The listing builds one solid part. Answer for the finished solid, in the listing's coordinates (mm). A direction names the side the tool comes from. Round coordinates to 2 decimals unless told otherwise and drop trailing zeros. Write each loop counter-clockwise with the first axis right and the second up, starting at its lowest first coordinate (ties: lowest second). Pieces come first, ordered by that corner, then holes.
(1) A cutting plane is placed at D-D, the plane y = -19.5. Give the vertices of the cut face in (x, z), and give its area (3 significant figures).
(2) A cutting plane is placed at B-B, the plane x = 25.5. Give the vertices of the cut face in (y, z).
(3) A cutting plane is placed at C-C, the plane z = 1159.5. Give the vertices of the cut face in (x, y).
(4) For faces 1 (the face through (-25.854, -14, 902)), 2 (the face through (16, -38.286, 902)), determine the directions among +Z, -Z, +X, -X, +Y, -Y from which every point of the face is accessible in a straight line to the end or side of a thin tool.
(5) Find the intervals of material crossed by probe 1 along Y at (x, z) = (26.5, 1719.5); probe 2 along X at (y, z) = (-18.5, 498); probe 3 along Y at (x, z) = (-15, 1494), in increasing order.
(6) Each of these flat-tipped pins is pushed along its axis until it touches: pin 1 Ø2 at (y, z) = (-11, 289.5) entering from +X; pin 2 Ø4 at (x, z) = (12, 508) entering from +Y; pin 3 Ø3 at (x, z) = (-23.5, 907.5) entering from +Y; pin 4 Ø5 at (x, y) = (-22, 27.5) entering from -Z. Where does it stop, or does it pass through?
(7) A cutting plane is placed at A-A, the plane z = 221. Give the vertices of the cut face in (x, y).
Autodesk Inventor part; units mm, degrees
ref_plane "YZ Plane" through (0, 0, 0) normal (1, 0, 0) x (0, 1, 0)
ref_plane "XZ Plane" through (0, 0, 0) normal (0, 1, 0) x (-1, 0, 0)
ref_plane "XY Plane" through (0, 0, 0) normal (0, 0, 1) x (1, 0, 0)
sketch "Sketch1" plane through (0, 0, 0) normal (0, 0, 1) x (1, 0, 0)
  line L0 (-25.8536, 31.5645) -> (-25.8536, -44.6355)
  line L1 (-25.8536, -44.6355) -> (50.3464, -44.6355)
  line L2 (50.3464, -44.6355) -> (50.3464, -44.1275)
  line L3 (44.5044, -38.2855) -> (-13.6616, -38.2855)
  line L4 (-19.5036, -32.4435) -> (-19.5036, 25.7225)
  line L5 (-25.3456, 31.5645) -> (-25.8536, 31.5645)
  arc A0 (50.3464, -44.1275) -> (44.5044, -38.2855) centre (44.5044, -44.1275) ccw
  arc A1 (-19.5036, 25.7225) -> (-25.3456, 31.5645) centre (-25.3456, 25.7225) ccw
  arc A2 (-19.5036, -32.4435) -> (-13.6616, -38.2855) centre (-13.6616, -32.4435) ccw
  point P0 (-19.5036, 31.5645)
  dimension "d0" = 76.2
  dimension "d1" = 76.2
  dimension "d2" = 6.35
  dimension "d3" = 5.842
extrude "Extrusion1" add sketch "Sketch1" along normal blind 1828.8
sketch "Sketch2" plane through (-25.8536, -44.6355, 0) normal (-1, 0, 0) x (0, 0, 1)
  line L0 (1828.8, 0) -> (1828.8, 76.2)
  line L1 (0, 76.2) -> (1828.8, 76.2)
  line L2 (0, 76.2) -> (0, 0)
  line L3 (0, 0) -> (1828.8, 0)
  line L4 (381, 76.2) -> (381, 63.5)
  line L5 (406.4, 38.1) -> (1422.4, 38.1)
  line L6 (1447.8, 63.5) -> (1447.8, 76.2)
  line L7 (1447.8, 76.2) -> (381, 76.2)
  arc A0 (381, 63.5) -> (406.4, 38.1) centre (406.4, 63.5) ccw
  arc A1 (1422.4, 38.1) -> (1447.8, 63.5) centre (1422.4, 63.5) ccw
  dimension "d6" = 25.4
  dimension "d7" = 38.1
  dimension "d8" = 381
  dimension "d9" = 381
extrude "Extrusion2" cut sketch "Sketch2" against normal mid plane 1828.8 contours L6 A1 L5 A0 L4 L1
properties part number "FE-00006-01"
Solutions:
1. outline: (-25.85, 0) - (-19.5, 0) - (-19.5, 1828.8) - (-25.85, 1828.8) - close
1. area: 11,600 mm2
2. outline: (-44.64, 0) - (-38.29, 0) - (-38.29, 1828.8) - (-44.64, 1828.8) - close
3. outline: (-25.85, -44.64) - (50.35, -44.64) - (50.35, -44.13) arc R5.84 ccw to (44.5, -38.29) - (-13.66, -38.29) arc R5.84 cw to (-19.5, -32.44) - (-19.5, -6.54) - (-25.85, -6.54) - close
4. face 1: +Z, -Z, -X, +Y, -Y
4. face 2: +Z, -Z, +X, +Y
5. probe 1: y = -44.64 to -38.29
5. probe 2: x = -25.85 to -19.5
5. probe 3: y = -44.64 to -38.13
6. pin 1: stops at x = -19.5
6. pin 2: stops at y = -38.29
6. pin 3: stops at y = -6.54
6. pin 4: stops at z = 0
7. outline: (-25.85, -44.64) - (50.35, -44.64) - (50.35, -44.13) arc R5.84 ccw to (44.5, -38.29) - (-13.66, -38.29) arc R5.84 cw to (-19.5, -32.44) - (-19.5, 25.72) arc R5.84 ccw to (-25.35, 31.56) - (-25.85, 31.56) - close
